Solid Edge part; units mm, degrees
sketch "Sketch1" plane through (0, 0, 0) normal (0, -1, 0) x (1, 0, 0)
  line L0 (154.74, 28) -> (0, 28)
  line L1 (0, 28) -> (0, 0)
  line L2 (0, 0) -> (154.74, 0)
  line L3 (154.74, 0) -> (154.74, 28)
extrude "Protrusion1" add sketch "Sketch1" against normal blind 4
sketch "Sketch2" plane through (77.37, 4, 14) normal (0, 1, 0) x (-1, 0, 0)
  line L0 (77.37, 14) -> (57.37, 14)
  line L1 (57.37, 14) -> (57.37, -14)
  line L2 (57.37, -14) -> (77.37, -14)
  line L3 (77.37, -14) -> (77.37, 14)
extrude "Recorte_Extrudado_3" cut sketch "Sketch2" against normal blind 2
sketch "Sketch3" plane through (77.37, 0, 14) normal (0, -1, 0) x (1, 0, 0)
  line L0 (77.37, -11) -> (-77.37, -11)
  line L1 (-77.37, -11) -> (-77.37, -14)
  line L2 (-77.37, -14) -> (77.37, -14)
  line L3 (77.37, -14) -> (77.37, -11)
extrude "Protrusão_Extrudada_4" add sketch "Sketch3" along normal blind 5
sketch "Sketch4" plane through (77.37, 0, 14) normal (0, -1, 0) x (1, 0, 0)
  line L0 (77.37, -11) -> (-77.37, -11)
  line L1 (-77.37, -11) -> (-77.37, -14)
  line L2 (-77.37, -14) -> (77.37, -14)
  line L3 (77.37, -14) -> (77.37, -11)
extrude "Protrusão_Extrudada_5" add sketch "Sketch4" against normal blind 19
Part model, mm, in its own coordinate system. A direction names the side the tool comes from. Round coordinates to 2 decimals unless told otherwise and drop trailing zeros. Write each loop counter-clockwise with the first axis right and the second up, starting at its lowest first coordinate (ties: lowest second). Pieces come first, ordered by that corner, then holes. Notation, with made-up numbers: (84, -14) -> (98, -14) arc R21 ccw to (98, -9) -> close; hole circle Ø5 at (79, 46). An arc over 180 degrees is marked (long way). Return JSON: item names as keys, results as strings. Group by question number.
Q1. Which spindle directions (+Z, -Z, +X, -X, +Y, -Y) get a long thin tool onto all of the face, cutting with end or side? Do faces 1 (the flat face through (78, -2, 3)), 2 (the flat face through (76, 7, 0)), 3 (the flat face through (88, 4, 16)), 4 (the flat face through (10, 2, 15)). Say none if no direction does.
Q2. Saw through at A-A on x = 16.5. Write the cut outline in (y, z).
Q3. Saw through at B-B on z = 19. Write the cut outline in (x, y).
Q4. Pin check, flat tips, straight feed: pin 1 (1 mm diameter, centred on y = 3.5, z = 17.5, fed in from -X); pin 2 (2 mm diameter, centred on x = 51, z = 10, fed in from -Y); pin 3 (12 mm diameter, centred on x = 23, z = 14, fed in from +Y). Stop position of each tip, or through.
Q5. Saw through at C-C on y = 7.25. Write the cut outline in (x, z).
Q6. Saw through at D-D on x = 128. Write the cut outline in (y, z).
Q7. Probe L1, parallel to Y at x = 119, z = 4.5; L2, parallel to Z at x = 66, y = 6; L3, parallel to X at y = 3, z = 15.5. List the from-to ranges inside material, lowest first. Write a range as [from, to].
Answer:
{
 "1": {"face 1": "+Z, +X, -X, -Y", "face 2": "-Z, +X, -X, +Y, -Y", "face 3": "+Z, +X, -X, +Y", "face 4": "+Z, -X, +Y"},
 "2": {"outline": "(-5, 0) -> (19, 0) -> (19, 3) -> (2, 3) -> (2, 28) -> (0, 28) -> (0, 3) -> (-5, 3) -> close"},
 "3": {"outline": "(0, 0) -> (154.74, 0) -> (154.74, 4) -> (20, 4) -> (20, 2) -> (0, 2) -> close"},
 "4": {"pin 1": "x = 20", "pin 2": "y = 0", "pin 3": "y = 4"},
 "5": {"outline": "(0, 0) -> (154.74, 0) -> (154.74, 3) -> (0, 3) -> close"},
 "6": {"outline": "(-5, 0) -> (19, 0) -> (19, 3) -> (4, 3) -> (4, 28) -> (0, 28) -> (0, 3) -> (-5, 3) -> close"},
 "7": {"L1": "[0, 4]", "L2": "[0, 3]", "L3": "[20, 154.74]"}
}
